Autodesk Inventor part; units mm, degrees
ref_plane "YZ Plane" through (0, 0, 0) normal (1, 0, 0) x (0, 1, 0)
ref_plane "XZ Plane" through (0, 0, 0) normal (0, 1, 0) x (-1, 0, 0)
ref_plane "XY Plane" through (0, 0, 0) normal (0, 0, 1) x (1, 0, 0)
sketch "Sketch8" plane through (0, 0, 0) normal (0, 0, 1) x (1, 0, 0)
  circle A0 centre (0, 0) radius 6.35
  line L0 (0, -153.4083) -> (0, 40.3847)
  line L1 (0, 12.7) -> (59.142, 12.7)
  line L2 (59.142, 12.7) -> (120.4631, -48.621)
  line L3 (120.4631, -48.621) -> (102.5026, -66.5815)
  line L4 (102.5026, -66.5815) -> (48.621, -12.7)
  line L5 (0, 0) -> (88.4811, -88.4811) construction
  line L6 (48.621, -12.7) -> (12.7, -48.621)
  line L7 (0, 12.7) -> (-59.142, 12.7)
  line L8 (-59.142, 12.7) -> (-120.4631, -48.621)
  line L9 (-120.4631, -48.621) -> (-102.5026, -66.5815)
  line L10 (-102.5026, -66.5815) -> (-48.621, -12.7)
  line L11 (0, 0) -> (-88.4811, -88.4811) construction
  line L12 (-48.621, -12.7) -> (-12.7, -48.621)
  line L13 (0, -71.842) -> (53.8815, -125.7236)
  line L14 (53.8815, -125.7236) -> (71.842, -107.7631)
  line L15 (71.842, -107.7631) -> (12.7, -48.621)
  line L16 (0, -71.842) -> (-53.8815, -125.7236)
  line L17 (-53.8815, -125.7236) -> (-71.842, -107.7631)
  line L18 (-71.842, -107.7631) -> (-12.7, -48.621)
  dimension "d108" = 12.7
  dimension "d110" = 25.4
  dimension "d111" = 76.2
  dimension "d112" = 12.7
  dimension "d113" = 12.7
  dimension "d114" = 50.8
  dimension "d115" = 135
  dimension "d131" = 76.2
  dimension "d133" = 25.4
extrude "Extrusion6" add sketch "Sketch8" along normal mid plane 3.175 contours A0 L0 L1 L2 L3 L4 L6 L15 L14 L13 | A0 L0 L16 L17 L18 L12 L10 L9 L8 L7
sketch "Sketch9" plane through (0, 0, 1.5875) normal (0, 0, 1) x (1, 0, 0)
  line L0 (-59.142, 12.7) -> (-120.4631, -48.621)
  line L1 (-102.5026, -66.5815) -> (-48.621, -12.7)
  line L2 (-120.4631, -66.5815) -> (0, 53.8815) construction
  line L3 (0, -161.6446) -> (0, 89.8026) construction
  circle A0 centre (-102.5026, -48.621) radius 2.65
  line L4 (-120.4631, -48.621) -> (-102.5026, -66.5815) construction
  circle A1 centre (-84.542, -30.6605) radius 2.65
  circle A2 centre (-66.5815, -12.7) radius 2.65
  line L5 (-93.5249, -93.5249) -> (0, 0) construction
  line L6 (-71.842, -125.7236) -> (0, -53.8815) construction
  line L7 (-12.7, -48.621) -> (-71.842, -107.7631) construction
  circle A3 centre (-53.8815, -107.7631) radius 2.65
  line L8 (-71.842, -107.7631) -> (-53.8815, -125.7236) construction
  circle A4 centre (-35.921, -89.8026) radius 2.65
  circle A5 centre (-17.9605, -71.842) radius 2.65
  dimension "d119" = 45
  dimension "d120" = 12.7
  dimension "d121" = 5.3
  dimension "d124" = 25.4
  dimension "d134" = 5.3
  dimension "d135" = 12.7
  dimension "d138" = 25.4
extrude "Extrusion7" cut sketch "Sketch9" against normal blind 25.4
mirror "Mirror3" about plane through (0, 0, 0) normal (1, 0, 0) of "Extrusion7"
fillet "Fillet4" radius 12.7 5 edges at (-48.621, -12.7, 0) (48.621, -12.7, 0) (0, -71.842, 0) (-12.7, -48.621, 0) (12.7, -48.621, 0)
equation "\"topDiameter\" = 45"
equation "\"bearingDiameter\" = 28.62"
equation "\"plateThickness\" = 6.35"
equation "\"theta12\" = 90deg"
equation "\"gearboxLength\" = 101.6"
equation "\"boltedLength\" = 76.2"
equation "\"topDiameter_1\" = 25"
equation "\"shaftLength_1\" = 76.2"
equation "\"bearingDiameter_1\" = 28.62"
equation "\"plateThickness_1\" = 6.35"
equation "\"theta12_1\" = 100deg"
equation "\"boltDiameter_1\" = 6"
equation "\"gearboxLength_1\" = 101.6"
equation "\"boltedLength_1\" = 76.2"
equation "\"innerBoltSpacing_1\" = 12.7"
equation "\"outerBoltSpacing_1\" = 12.7"
equation "\"shaftLength\" = 76.2"
equation "\"boltDiameter\" = 5.3"
equation "\"outerBoltSpacing\" = 12.7"
equation "\"innerBoltSpacing\" = 12.7"
properties part number "KneePivotPlate" material "Aluminum 6061"
For this review, take the finished solid that the model builds, in its own axes (mm). A direction names the side the tool comes from. Round coordinates to 2 decimals unless told otherwise and drop trailing zeros. Loops run counter-clockwise (first coordinate to the right, second up) from the corner with the lowest first, then second, coordinate; pieces in that order, holes last. Notation, with made-up numbers: (86, 82) - (118, 82) arc R30 cw to (118, 116) - close; hole circle Ø4 at (86, -8). An arc over 180 degrees is marked (long way). Answer as CSV lines item,"result".
(1) Consider section D-D on y = -12.7. Give the boundary of the cut face in (x, z).
Checked values:
outline,"(-84.54, -1.59) - (-69.23, -1.59) - (-69.23, 1.59) - (-84.54, 1.59) - close; (-63.93, -1.59) - (63.93, -1.59) - (63.93, 1.59) - (-63.93, 1.59) - close; (69.23, -1.59) - (84.54, -1.59) - (84.54, 1.59) - (69.23, 1.59) - close"
(2) Insertion check: P1, Ø1, axis at y = -108.5, z = 0.5, coming from the +X side; P2, Ø3, axis at x = 84.54, y = -30.66, coming from the -Z side; P3, Ø8.5, axis at x = 102.5, y = -48.62, coming from the +Z side. Each pin has a flat end and moves straight along its axis. Give the tip position at first contact, or say it passes through.
Checked values:
P1,"stops at x = 71.61"
P2,"passes through"
P3,"stops at z = 1.59"
(3) Consider section B-B on y = -95.5. Give the boundary of the cut face in (x, z).
Checked values:
outline,"(-59.58, -1.59) - (-23.66, -1.59) - (-23.66, 1.59) - (-59.58, 1.59) - close; (23.66, -1.59) - (59.58, -1.59) - (59.58, 1.59) - (23.66, 1.59) - close"
(4) Consider section A-A on x = 0. Give the boundary of the cut face in (y, z).
Checked values:
outline,"(-77.1, -1.59) - (-6.35, -1.59) - (-6.35, 1.59) - (-77.1, 1.59) - close; (6.35, -1.59) - (12.7, -1.59) - (12.7, 1.59) - (6.35, 1.59) - close"
(5) Tool access review of faces 1 (the face through (47.11, -83.03, 0.02)), 2 (the face through (-111.609, -57.476, 0.022)), 3 (the face through (31.12, -102.96, 0.02)): name each direction out of +Z, -Z, +X, -X, +Y, -Y from which nothing blocks a thin tool from reaching the whole face with its end or side.
Checked values:
face 1,"+Z, -Z"
face 2,"+Z, -Z, -X, -Y"
face 3,"+Z, -Z, -Y"
(6) Consider section C-C on z = -0.9. Give the number of separate pieces and of enclosed holes in the cut face, then the cut area to 3 significant figures.
Checked values:
separate pieces,"1"
enclosed holes,"13"
area,"13,200 mm2"
(7) Wall thickness on line 1 (X direction, y = -57, z = 1); line 2 (X direction, y = 0, z = 0.05); line 3 (X direction, y = -42.5, z = -1.15): over which ranges is each line inside the solid? List them lowest first.
Checked values:
line 1,"x = -112.08 to -92.92, -21.12 to 21.12, 92.92 to 112.08"
line 2,"x = -71.84 to -6.35, 6.35 to 71.84"
line 3,"x = -114.34 to -78.42, -19.53 to 19.53, 78.42 to 114.34"
(8) Mouldability with a two-part tool opening along Y and no side actions: class faces 4 (the face through (-31.12, -102.96, 0.02)), 5 (the face through (89.37, -17.53, 0.02)), 6 (the face through (-68.535, -10.909, 0.022)), 7 (the face through (-2, -40, -1.588)) as +Y half, -Y half, draft (parallel to the pull), parting line (faces both ways), or undercut.
Checked values:
face 4,"-Y half"
face 5,"+Y half"
face 6,"undercut"
face 7,"draft"
